Build history of the part. All positions in model axes, mm. Give positions to 0.01 mm unless a question says otherwise; leave off trailing zeros. Write each loop counter-clockwise with the first axis right and the second up, starting at its lowest first coordinate (ties: lowest second). Pieces come first, ordered by that corner, then holes. Notation, with made-up numbers: (69.5, -34) - (109.5, -34) arc R19 ccw to (109.5, 0) - close; hole circle Ø7 at (63, -38.75). An arc over 180 degrees is marked (long way). Use one line per item in the form item = value. Start each with the question number.
from build123d import *


with BuildPart() as f1:
    # F0 (on Front) → F1 (revolve)
    with BuildSketch(Plane.XZ):
        with BuildLine():
            Line((0, 8.382), (0, 0))
            Line((0, 0), (1.905, 0))
            Line((1.905, 0), (1.905, 8.382))
            ThreePointArc((1.905, 8.382), (3.3557, 11.8843), (6.858, 13.335))
            Line((6.858, 13.335), (281.686, 13.335))
            Line((281.686, 13.335), (281.686, 15.24))
            Line((281.686, 15.24), (23.494648, 15.24))
            Line((23.494648, 15.24), (6.858, 15.24))
            ThreePointArc((6.858, 15.24), (2.008662, 13.231338), (0, 8.382))
        make_face()
    revolve(axis=Axis((281.686, 0, 14.2875), (0, 0, 1)))


solid = f1.part
(1) Cut at A-A, the plane y = 0. Give the cut face in (x, z) (3 decimals).
(2) Two-plate mould, pull along X, no slides. Class faces 1 (the flat face through (286, -4, 13.335)), 2 (the flat face through (278, -4, 15.24)), 3 (the cylindrical face through (14.825, -84.039, 4.25)), 4 (the cylindrical face through (563.1, -12.4, 4.1)): +X half, -X half, draft (parallel to the pull), parting line (faces both ways), or undercut.
(3) Wall check: line 1 (Y direction, x = 290, z = 3); line 2 (X direction, y = 0, z = 2) (3 decimals); line 3 (Z direction, x = 484.5, y = 186). Give the ranges that are in metal, low to high. Write a range as from..to.
(4) Pin check, flat tips, straight feed: pin 1 Ø8 at (y, z) = (-154.5, 6) entering from -X; pin 2 Ø4 at (y, z) = (-192, 1.5) entering from +X; pin 3 Ø3 at (y, z) = (17.5, 8) entering from +X. Stop position of each tip, or through.
Solution:
q1.outline = (0, 0) - (1.905, 0) - (1.905, 8.382) arc R4.953 cw to (6.858, 13.335) - (556.514, 13.335) arc R4.953 cw to (561.467, 8.382) - (561.467, 0) - (563.372, 0) - (563.372, 8.382) arc R6.858 ccw to (556.514, 15.24) - (6.858, 15.24) arc R6.858 ccw to (0, 8.382) - close
q2.face_1 = undercut
q2.face_2 = draft
q2.face_3 = undercut
q2.face_4 = parting line
q3.line_1 = -281.56..-279.66, 279.66..281.56
q3.line_2 = 0..1.905, 561.467..563.372
q3.line_3 = 13.32..15.23
q4.pin_1 = 43.58
q4.pin_2 = 489.65
q4.pin_3 = 562.92
